Design review of the part shown in the three views and the two pictorial views. Dimensions are in mm from the part's minimum x, y and z. A direction names the side the tool comes from. Round coordinates to 2 decimals unless told otherwise and drop trailing zeros. Write each loop counter-clockwise with the first axis right and the second up, starting at its lowest first coordinate (ties: lowest second). Pieces come first, ordered by that corner, then holes. Notation, with made-up numbers: (26, 44) - (85, 44) arc R18 ccw to (85, 59) - close; hole circle Ø1 at (-0.75, -29). An arc over 180 degrees is marked (long way). Use one line per item in the form item = value.
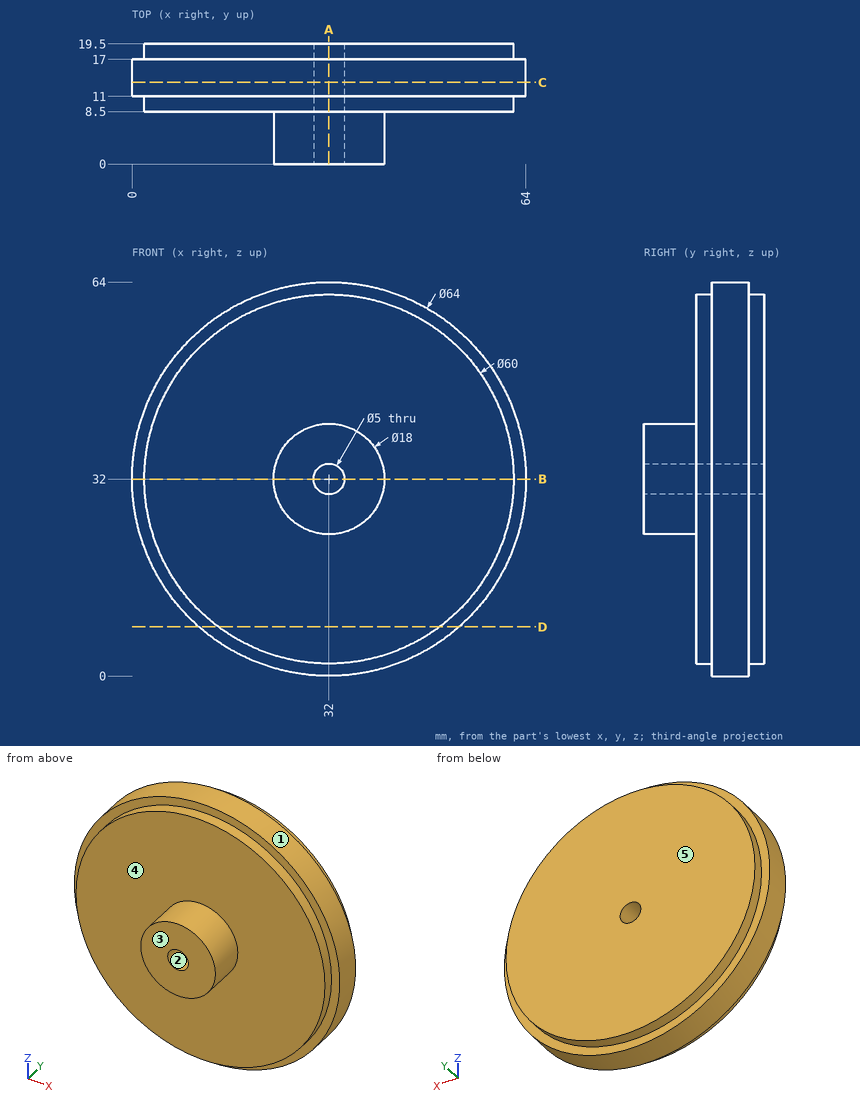
(1) Add section C-C on y = 13.25. Write out the cut boundary in (x, z).
Geometry results:
outline = circle Ø64 at (32, 32); hole circle Ø5 at (32, 32)
(2) The part is to be moulded in two halves that separate along X. For the marked faces 1, 2 and 3, say which applies: +X half, -X half, draft (parallel to the pull), parting line (faces both ways), or undercut.
Geometry results:
face_1 = parting line
face_2 = undercut
face_3 = draft
(3) Machinability: for the marked faces 4 and 5, which of the approach directions +Z, -Z, +X, -X, +Y, -Y give a long, thin tool a straight path to every point of the face, cutting with its end or side? Answer none if there is none.
Geometry results:
face_4 = -Y
face_5 = +Z, -Z, +X, -X, +Y
(4) To check wall thickness, follow L1, parallel to X at y = 14.5, z = 32; L2, parallel to X at y = 10.75, z = 32; L3, parallel to Z at x = 31, y = 15. State the ranges of each line that lie inside material, in increasing order.
Geometry results:
L1 = 0 to 29.5, 34.5 to 64
L2 = 2 to 29.5, 34.5 to 62
L3 = 0.02 to 29.71, 34.29 to 63.98
(5) Insertion check: P1, Ø8, axis at x = 41, z = 41.5, coming from the -Y side; P2, Ø10, axis at x = 37.5, y = 11, coming from the -Z side; P3, Ø8, axis at x = 27.5, y = 11, coming from the +Z side. Each pin has a flat end and moves straight along its axis. Give the tip position at first contact, or say it passes through.
Geometry results:
P1 = 8.5
P2 = 0
P3 = 64
(6) Add section B-B on z = 32. Write out the cut boundary in (x, y).
Geometry results:
outline = (0, 11) - (2, 11) - (2, 8.5) - (23, 8.5) - (23, 0) - (29.5, 0) - (29.5, 19.5) - (2, 19.5) - (2, 17) - (0, 17) - close; (34.5, 0) - (41, 0) - (41, 8.5) - (62, 8.5) - (62, 11) - (64, 11) - (64, 17) - (62, 17) - (62, 19.5) - (34.5, 19.5) - close
(7) Add section D-D on z = 8. Write out the cut boundary in (x, y).
Geometry results:
outline = (10.83, 11) - (14, 11) - (14, 8.5) - (50, 8.5) - (50, 11) - (53.17, 11) - (53.17, 17) - (50, 17) - (50, 19.5) - (14, 19.5) - (14, 17) - (10.83, 17) - close
(8) Add section A-A on x = 32. Write out the cut boundary in (y, z).
Geometry results:
outline = (0, 23) - (8.5, 23) - (8.5, 2) - (11, 2) - (11, 0) - (17, 0) - (17, 2) - (19.5, 2) - (19.5, 29.5) - (0, 29.5) - close; (0, 34.5) - (19.5, 34.5) - (19.5, 62) - (17, 62) - (17, 64) - (11, 64) - (11, 62) - (8.5, 62) - (8.5, 41) - (0, 41) - close
